Answer from the drawing. Dimensions are ordinates in mm from the lowest x, y and z of the part. A direction names the side the tool comes from. Give positions to 0.01 mm unless a question says otherwise; leave off trailing zeros. Order: outer loops, then holes, each group sorted by start corner. A loop starts at its lowest first (then second) coordinate and runs counter-clockwise, first axis right, second up. Notation, with made-up numbers: (-35.75, 89.5) - (7.25, 89.5) arc R32 ccw to (7.25, 124.5) - close; hole circle Ø3 at (34, 82). An arc over 180 degrees is marked (long way). Answer in a Markdown table with one row per item. Add a question column.
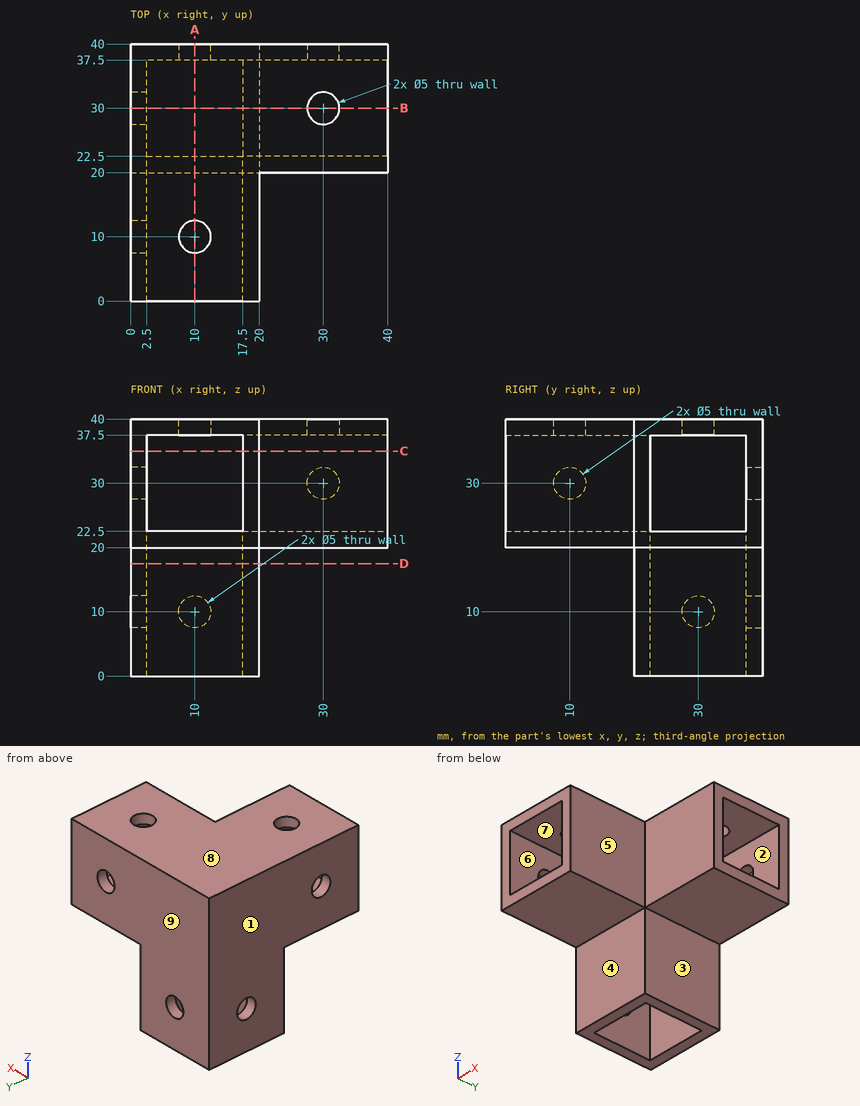
(1) Straight lines are drawn through the part: line 1 (X direction, y = 9.5, z = 37); line 2 (Y direction, x = 30, z = 38); line 3 (Y direction, x = 33.5, z = 33.5). For each, find the intervals that lie inside material, in ascending order.
(2) Find section C-C, the plane z = 35. Write down the section's boundary in (x, y), plus the area to 3 significant figures.
(3) Find section D-D, the plane z = 17.5. Write down the section's boundary in (x, y), plus the area to 3 significant figures.
(4) Find section A-A, the plane x = 10. Write down the section's boundary in (y, z), plus the area to 3 significant figures.
(5) The mould has two halves that part along Z. Classify the marked faces 6, 7, 8 and 9: +Z half, -Z half, draft (parallel to the pull), parting line (faces both ways), or undercut.
(6) Each of these flat-tipped pins is pushed along its axis until it touches: P1, Ø22, axis at x = 32, y = 28.5, coming from the -Z side; P2, Ø1.5, axis at y = 32, z = 5, coming from the +X side; P3, Ø10, axis at x = 26.5, z = 29, coming from the -Y side. Where does it stop, or does it pass through?
(7) For the marked faces 1, 2, 3, 4 and 5, determine the directions among +Z, -Z, +X, -X, +Y, -Y from which every point of the face is accessible in a straight line to the end or side of a thin tool.
(8) Find section B-B, the plane y = 30. Write down the section's boundary in (x, z), plus the area to 3 significant figures.
Answer key:
| question | item | result |
|---|---|---|
| 1 | line 1 | 0 to 2.5, 17.5 to 20 |
| 1 | line 2 | 20 to 27.5, 32.5 to 40 |
| 1 | line 3 | 20 to 22.5, 37.5 to 40 |
| 2 | outline | (0, 0) - (2.5, 0) - (2.5, 37.5) - (40, 37.5) - (40, 40) - (0, 40) - close; (17.5, 0) - (20, 0) - (20, 20) - (40, 20) - (40, 22.5) - (17.5, 22.5) - close |
| 2 | area | 300 mm² |
| 3 | outline | (0, 20) - (20, 20) - (20, 40) - (0, 40) - close; hole (2.5, 22.5) - (17.5, 22.5) - (17.5, 37.5) - (2.5, 37.5) - close |
| 3 | area | 175 mm² |
| 4 | outline | (0, 20) - (20, 20) - (20, 0) - (22.5, 0) - (22.5, 22.5) - (0, 22.5) - close; (0, 37.5) - (7.5, 37.5) - (7.5, 40) - (0, 40) - close; (12.5, 37.5) - (37.5, 37.5) - (37.5, 12.5) - (40, 12.5) - (40, 40) - (12.5, 40) - close; (37.5, 0) - (40, 0) - (40, 7.5) - (37.5, 7.5) - close |
| 4 | area | 275 mm² |
| 5 | face 6 | undercut |
| 5 | face 7 | undercut |
| 5 | face 8 | +Z half |
| 5 | face 9 | draft |
| 6 | P1 | z = 20 |
| 6 | P2 | x = 20 |
| 6 | P3 | y = 20 |
| 7 | face 1 | +Z, -Z, -X, +Y, -Y |
| 7 | face 2 | none |
| 7 | face 3 | -Z, +X, +Y, -Y |
| 7 | face 4 | -Z, +X, -X, -Y |
| 7 | face 5 | +Z, -Z, +X, -Y |
| 8 | outline | (0, 0) - (2.5, 0) - (2.5, 7.5) - (0, 7.5) - close; (0, 12.5) - (2.5, 12.5) - (2.5, 37.5) - (27.5, 37.5) - (27.5, 40) - (0, 40) - close; (17.5, 0) - (20, 0) - (20, 20) - (40, 20) - (40, 22.5) - (17.5, 22.5) - close; (32.5, 37.5) - (40, 37.5) - (40, 40) - (32.5, 40) - close |
| 8 | area | 275 mm² |
